from build123d import *

# Parameters (mm, degrees)
CUT_EXTRUDE1_START       = -13
CUT_EXTRUDE1_OUTLINE_R   = 14.975
CUT_EXTRUDE1_OUTLINE_R_2 = 3.125
CUT_EXTRUDE1_DEPTH       = 13
CUT_EXTRUDE1_START_2     = -8
CUT_EXTRUDE1_2_OUTLINE_R = 2
CUT_EXTRUDE1_2_DEPTH     = 8
CUT_EXTRUDE3_DEPTH       = 5
BOSS_EXTRUDE1_DEPTH      = 13
CUT_EXTRUDE4_DEPTH       = 2
CUT_EXTRUDE4_DEPTH_BACK  = 22
BOSS_EXTRUDE2_REACH      = 26.85


with BuildPart() as part:
    # Cut-Extrude1: read off the stored shape, not the designer's step
    # Cut-Extrude1 outline → Cut-Extrude1 (new body)
    with BuildSketch(Plane.XY.offset(13).offset(CUT_EXTRUDE1_START)):
        Circle(CUT_EXTRUDE1_OUTLINE_R)
        Polygon((-6.363961031, -2.380244173), (-2.913961031, -4.372102602), (-2.913961031, -8.355819459), (-6.363961031, -10.347677888), (-9.813961031, -8.355819459), (-9.813961031, -4.372102602), align=None, mode=Mode.SUBTRACT)
        Polygon((9.813961031, -8.355819459), (6.363961031, -10.347677888), (2.913961031, -8.355819459), (2.913961031, -4.372102602), (6.363961031, -2.380244173), (9.813961031, -4.372102602), align=None, mode=Mode.SUBTRACT)
        Circle(CUT_EXTRUDE1_OUTLINE_R_2, mode=Mode.SUBTRACT)
        Polygon((-9.813961031, 8.355819459), (-6.363961031, 10.347677888), (-2.913961031, 8.355819459), (-2.913961031, 4.372102602), (-6.363961031, 2.380244173), (-9.813961031, 4.372102602), align=None, mode=Mode.SUBTRACT)
        Polygon((6.363961031, 2.380244173), (2.913961031, 4.372102602), (2.913961031, 8.355819459), (6.363961031, 10.347677888), (9.813961031, 8.355819459), (9.813961031, 4.372102602), align=None, mode=Mode.SUBTRACT)
    extrude(amount=CUT_EXTRUDE1_DEPTH)

    # Cut-Extrude1 2 outline → Cut-Extrude1 2 (add)
    # profile 1 of 4: a face of its own
    with BuildSketch(Plane.XY.offset(13).offset(CUT_EXTRUDE1_START_2)):
        Polygon((2.913961031, -8.355819459), (6.363961031, -10.347677888), (9.813961031, -8.355819459), (9.813961031, -4.372102602), (6.363961031, -2.380244173), (2.913961031, -4.372102602), align=None)
        with Locations((6.363961031, -6.363961031)):
            Circle(CUT_EXTRUDE1_2_OUTLINE_R, mode=Mode.SUBTRACT)
    # profile 2 of 4: a face of its own
    with BuildSketch(Plane.XY.offset(13).offset(CUT_EXTRUDE1_START_2)):
        Polygon((-2.913961031, -8.355819459), (-2.913961031, -4.372102602), (-6.363961031, -2.380244173), (-9.813961031, -4.372102602), (-9.813961031, -8.355819459), (-6.363961031, -10.347677888), align=None)
        with Locations((-6.363961031, -6.363961031)):
            Circle(CUT_EXTRUDE1_2_OUTLINE_R, mode=Mode.SUBTRACT)
    # profile 3 of 4: a face of its own
    with BuildSketch(Plane.XY.offset(13).offset(CUT_EXTRUDE1_START_2)):
        Polygon((-2.913961031, 8.355819459), (-6.363961031, 10.347677888), (-9.813961031, 8.355819459), (-9.813961031, 4.372102602), (-6.363961031, 2.380244173), (-2.913961031, 4.372102602), align=None)
        with Locations((-6.363961031, 6.363961031)):
            Circle(CUT_EXTRUDE1_2_OUTLINE_R, mode=Mode.SUBTRACT)
    # profile 4 of 4: a face of its own
    with BuildSketch(Plane.XY.offset(13).offset(CUT_EXTRUDE1_START_2)):
        Polygon((2.913961031, 8.355819459), (2.913961031, 4.372102602), (6.363961031, 2.380244173), (9.813961031, 4.372102602), (9.813961031, 8.355819459), (6.363961031, 10.347677888), align=None)
        with Locations((6.363961031, 6.363961031)):
            Circle(CUT_EXTRUDE1_2_OUTLINE_R, mode=Mode.SUBTRACT)
    extrude(amount=CUT_EXTRUDE1_2_DEPTH)

    # Cut-Extrude1 3: loft between two sections, ruled curve by curve
    cut_extrude1_3_from = [
        Edge.make_three_point_arc((0, 14.975, 1.45), (1.449568901, 14.975, 2.050431099), (2.05, 14.975, 3.5)),
        Edge.make_three_point_arc((2.05, 14.975, 3.5), (1.449568901, 14.975, 4.949568901), (0, 14.975, 5.55)),
        Edge.make_three_point_arc((0, 14.975, 5.55), (-1.449568901, 14.975, 4.949568901), (-2.05, 14.975, 3.5)),
        Edge.make_three_point_arc((-2.05, 14.975, 3.5), (-1.449568901, 14.975, 2.050431099), (0, 14.975, 1.45)),
    ]
    cut_extrude1_3_to = [
        Edge.make_three_point_arc((0, 2.358384549, 1.45), (1.449568901, 2.358384549, 2.050431099), (2.05, 2.358384549, 3.5)),
        Edge.make_three_point_arc((2.05, 2.358384549, 3.5), (1.449568901, 2.358384549, 4.949568901), (0, 2.358384549, 5.55)),
        Edge.make_three_point_arc((0, 2.358384549, 5.55), (-1.449568901, 2.358384549, 4.949568901), (-2.05, 2.358384549, 3.5)),
        Edge.make_three_point_arc((-2.05, 2.358384549, 3.5), (-1.449568901, 2.358384549, 2.050431099), (0, 2.358384549, 1.45)),
    ]
    cut_extrude1_3 = Solid(Shell([*[Face.make_surface_from_curves(cut_extrude1_3_from[k], cut_extrude1_3_to[k]) for k in range(4)], Face(Wire(cut_extrude1_3_from)), Face(Wire(cut_extrude1_3_to))]))
    add(cut_extrude1_3, mode=Mode.SUBTRACT)

    # Cut-Extrude1 4: loft between two sections, ruled curve by curve
    cut_extrude1_4_from = [
        Edge.make_three_point_arc((0, 14.975, 7.45), (1.449568901, 14.975, 8.050431099), (2.05, 14.975, 9.5)),
        Edge.make_three_point_arc((2.05, 14.975, 9.5), (1.449568901, 14.975, 10.949568901), (0, 14.975, 11.55)),
        Edge.make_three_point_arc((0, 14.975, 11.55), (-1.449568901, 14.975, 10.949568901), (-2.05, 14.975, 9.5)),
        Edge.make_three_point_arc((-2.05, 14.975, 9.5), (-1.449568901, 14.975, 8.050431099), (0, 14.975, 7.45)),
    ]
    cut_extrude1_4_to = [
        Edge.make_three_point_arc((0, 2.358384549, 7.45), (1.449568901, 2.358384549, 8.050431099), (2.05, 2.358384549, 9.5)),
        Edge.make_three_point_arc((2.05, 2.358384549, 9.5), (1.449568901, 2.358384549, 10.949568901), (0, 2.358384549, 11.55)),
        Edge.make_three_point_arc((0, 2.358384549, 11.55), (-1.449568901, 2.358384549, 10.949568901), (-2.05, 2.358384549, 9.5)),
        Edge.make_three_point_arc((-2.05, 2.358384549, 9.5), (-1.449568901, 2.358384549, 8.050431099), (0, 2.358384549, 7.45)),
    ]
    cut_extrude1_4 = Solid(Shell([*[Face.make_surface_from_curves(cut_extrude1_4_from[k], cut_extrude1_4_to[k]) for k in range(4)], Face(Wire(cut_extrude1_4_from)), Face(Wire(cut_extrude1_4_to))]))
    add(cut_extrude1_4, mode=Mode.SUBTRACT)

    # Sketch2 → Cut-Extrude3 (cut)
    with BuildSketch(Plane(origin=(0, 0, 0), x_dir=(-1, 0, 0), z_dir=(0, 0, -1))):
        Polygon((2.813961031, 8.413554486), (2.813961031, 4.314367575), (6.363961031, 2.264774119), (9.913961031, 4.314367575), (9.913961031, 8.413554486), (6.363961031, 10.463147942), align=None)
    extrude(amount=-CUT_EXTRUDE3_DEPTH, mode=Mode.SUBTRACT)

    # Sketch4 → Boss-Extrude1 (add)
    with BuildSketch(Plane(origin=(0, 0, 0), x_dir=(-1, 0, 0), z_dir=(0, 0, -1))):
        with BuildLine():
            ThreePointArc((-2.461706725, -1.925), (-1.369306394, -2.809025632), (0, -3.125))
            Line((0, -3.125), (0, -1.925))
            Line((0, -1.925), (-2.461706725, -1.925))
        make_face()
        with BuildLine():
            Line((0, -1.925), (0, -3.125))
            ThreePointArc((0, -3.125), (1.369306394, -2.809025632), (2.461706725, -1.925))
            Line((2.461706725, -1.925), (0, -1.925))
        make_face()
    extrude(amount=-BOSS_EXTRUDE1_DEPTH)

    # Sketch3 → Cut-Extrude4 (cut, two sides: drawn at the far end of the back side and taken through both)
    with BuildSketch(Plane(origin=(0, 0, 0), x_dir=(1, 0, 0), z_dir=(0, 1, 0)).offset(-CUT_EXTRUDE4_DEPTH_BACK)):
        with BuildLine():
            ThreePointArc((0, -4.5), (-1.5, -6), (0, -7.5))
            Line((0, -7.5), (0, -4.5))
        make_face()
        with BuildLine():
            Line((0, -4.5), (0, -7.5))
            ThreePointArc((0, -7.5), (1.060660172, -7.060660172), (1.5, -6))
            ThreePointArc((1.5, -6), (1.060660172, -4.939339828), (0, -4.5))
        make_face()
        with BuildLine():
            ThreePointArc((0, -9.350905038), (-1.25, -10.600905038), (0, -11.850905038))
            Line((0, -11.850905038), (0, -9.350905038))
        make_face()
        with BuildLine():
            Line((0, -9.350905038), (0, -11.850905038))
            ThreePointArc((0, -11.850905038), (0.883883476, -11.484788515), (1.25, -10.600905038))
            ThreePointArc((1.25, -10.600905038), (0.883883476, -9.717021562), (0, -9.350905038))
        make_face()
    extrude(amount=CUT_EXTRUDE4_DEPTH + CUT_EXTRUDE4_DEPTH_BACK, mode=Mode.SUBTRACT)

    # Sketch5 → Boss-Extrude2 (add, up to next)
    with BuildSketch(Plane(origin=(0, 0, 0), x_dir=(-1, 0, 0), z_dir=(0, 0, -1)), mode=Mode.PRIVATE) as boss_extrude2_sk1:
        with BuildLine():
            Line((-4.568894393, 14.260989763), (-3.6536631, 9.845398343))
            Line((-3.6536631, 9.845398343), (-2.698785597, 9.845398343))
            Line((-2.698785597, 9.845398343), (-2.04137138, 2.366099721))
            ThreePointArc((-2.04137138, 2.366099721), (0, 3.125), (2.04137138, 2.366099721))
            Line((2.04137138, 2.366099721), (2.335168556, 11.338349863))
            Line((2.335168556, 11.338349863), (6.630079619, 11.338349863))
            Line((6.630079619, 11.338349863), (8.4371537, 9.779282306))
            Line((8.4371537, 9.779282306), (9.782251652, 11.338349863))
            ThreePointArc((9.782251652, 11.338349863), (2.988348955, 14.673799628), (-4.568894393, 14.260989763))
        make_face()
    boss_extrude2_tool1 = extrude(boss_extrude2_sk1.sketch, amount=-BOSS_EXTRUDE2_REACH, mode=Mode.PRIVATE) - part.part
    add(boss_extrude2_tool1.solids().sort_by_distance((-0.855715, 10.107885, 0))[0])
    add(boss_extrude2_tool1.solids().sort_by_distance((-0.855715, 10.107885, 0))[1])


solid = part.part
CAD build for the part. Positions are in the model's coordinates, mm. A direction names the side the tool comes from. Coordinates: 2 decimals unless noted, no trailing zeros. Write each loop counter-clockwise with the first axis right and the second up, starting at its lowest first coordinate (ties: lowest second). Pieces come first, ordered by that corner, then holes. Notation, with made-up numbers: M 64.5,8 L 86.5,8 A15 cw 86.5,12 Z; hole C -14.75,38 d10. An arc over 180 degrees is marked long. Return JSON: item names as keys, results as strings.
Item 1: Slice it at A-A, the plane y = -5.25. Write the cut outline in (x, z).
Findings below:
{"outline": "M -14.02,0 L -9.81,0 L -9.81,5 L -8.03,5 L -8.03,13 L -14.02,13 Z; M -4.7,5 L -2.91,5 L -2.91,0 L 2.91,0 L 2.91,5 L 4.7,5 L 4.7,13 L -4.7,13 Z; M 8.03,5 L 9.81,5 L 9.81,0 L 14.02,0 L 14.02,13 L 8.03,13 Z; hole C 0,6 d3; hole C 0,10.6 d2.5"}
Item 2: Slice it at B-B, the plane x = 8. Write the cut outline in (y, z), and give its area (3 significant figures).
Findings below:
{"outline": "M -12.66,0 L -9.4,0 L -9.4,5 L -7.51,5 L -7.51,13 L -12.66,13 Z; M -5.21,5 L -3.32,5 L -3.32,0 L 3.32,0 L 3.32,5 L 5.21,5 L 5.21,13 L -5.21,13 Z; M 7.51,5 L 9.4,5 L 9.4,0 L 12.66,0 L 12.66,13 L 7.51,13 Z", "area": "232 mm2"}
Item 3: Slice it at C-C, the plane y = 8. Write the cut outline in (x, z).
Findings below:
{"outline": "M -12.66,0 L -9.91,0 L -9.91,5 L -7.51,5 L -7.51,13 L -12.66,13 Z; M -5.21,5 L -2.81,5 L -2.81,0 L 2.91,0 L 2.91,5 L 5.21,5 L 5.21,13 L -5.21,13 Z; M 7.51,5 L 9.81,5 L 9.81,0 L 12.66,0 L 12.66,13 L 7.51,13 Z"}
Item 4: Slice it at D-D, the plane y = -8.75. Write the cut outline in (x, z).
Findings below:
{"outline": "M -12.15,0 L -9.13,0 L -9.13,5 L -3.6,5 L -3.6,0 L 3.6,0 L 3.6,5 L 9.13,5 L 9.13,0 L 12.15,0 L 12.15,13 L -12.15,13 Z; hole C 0,6 d3; hole C 0,10.6 d2.5"}
Item 5: Two-plate mould, pull along X, no slides. Class faces 1 (the flat face through (9.814, -6, 2)), 2 (the flat face through (0, -3, 0)): +X half, -X half, draft (parallel to the pull), parting line (faces both ways), or undercut.
Findings below:
{"face 1": "undercut", "face 2": "draft"}
Item 6: Probe line 1 (X direction, y = -9, z = 2.25); line 2 (Y direction, x = 7.75, z = 12); line 3 (X direction, y = 6.75, z = 0.5). List the from-to ranges inside material, lowest first. Write a range as from..to.
Findings below:
{"line 1": "x = -11.97..-8.7, -4.03..4.03, 8.7..11.97", "line 2": "y = -12.81..-7.81, -4.92..4.92, 7.81..12.81", "line 3": "x = -13.37..-9.91, -2.81..2.91, 9.81..13.37"}
Item 7: Which spindle directions (+Z, -Z, +X, -X, +Y, -Y) get a long thin tool onto all of the face, cutting with end or side? Do faces 3 (the flat face through (-8.164, 9.424, 2.465)), 4 (the cylindrical face through (-8.362, -6.276, 8.944)). Say none if no direction does.
Findings below:
{"face 3": "-Z", "face 4": "+Z, -Z"}
Item 8: Drop flat-ended pins along their axis: pin 1 Ø3.5 at (y, z) = (5.5, 1.5) entering from -X; pin 2 Ø2 at (y, z) = (-11.5, 1.5) entering from -X; pin 3 Ø1 at (y, z) = (5, 3.5) entering from +X. Give the stop position or say it passes through.
Findings below:
{"pin 1": "stops at x = -14.5", "pin 2": "stops at x = -10.68", "pin 3": "stops at x = 14.28"}
